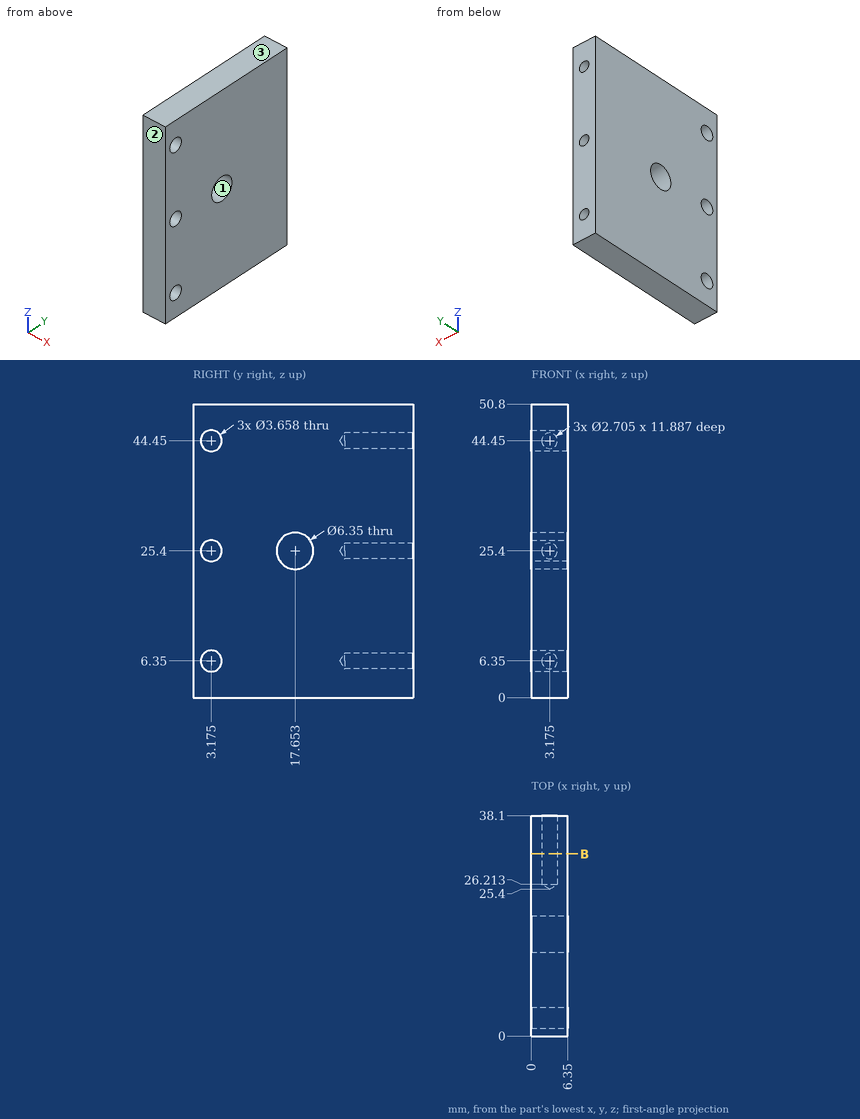
Check sheet for the drawn part. Datum: minimum x, y, z corner. Units: mm. Give positions to 0.01 mm unless a question says otherwise; leave off trailing zeros. One line per item, written item: value.
(1) Sectioned sample at B-B on y = 31.5. Count the separate pieces of the cut face and the enclosed holes in it, then the cut area to 3 significant figures.
Final values:
separate pieces: 1
enclosed holes: 3
area: 305 mm^2
(2) Scan lines: line 1 along X through (y, z) = (31, 25.4); line 2 along Y through (x, z) = (2.5, 25.4) (1 decimal); line 3 along Y through (x, z) = (1.5, 44.45). Record each from-to range of solid material in increasing order. Write a range as [from, to].
Final values:
line 1: [0, 1.82], [4.53, 6.35]
line 2: [0, 1.3], [5, 14.5], [20.8, 25.8]
line 3: [0, 1.35], [5, 38.1]
(3) Draft check along Y on the marked faces 1, 2 and 3. Enter one of: pulls with the +Y half, pulls with the -Y half, needs draft (parallel to the pull), parting line crosses it, or undercut.
Final values:
face 1: undercut
face 2: pulls with the -Y half
face 3: needs draft
(4) Gauge pin test, flat end, axial feed: pin 1 (2 mm diameter, centred on y = 3.175, z = 6.35, fed in from +X). Record the tip position at first contact, or that the pin passes through.
Final values:
pin 1: through
